Geometry check sheet. Reference: the model listing, model coordinates, mm. A direction names the side the tool comes from. Give positions to 0.01 mm unless a question says otherwise; leave off trailing zeros. Order: outer loops, then holes, each group sorted by start corner. A loop starts at its lowest first (then second) coordinate and runs counter-clockwise, first axis right, second up.
```python
from build123d import *

# Parameters (mm, degrees)
F2_T     = -1
F3_R     = 9.75
F4_DEPTH = 1


with BuildPart() as f1:
    # F0 (on Front) → F1 (revolve)
    with BuildSketch(Plane.XZ):
        Polygon((0, 12), (0, 0), (25, 0), (25, 8), (12.5, 12), align=None)
    revolve(axis=Axis((0, 0, 39.176005), (0, 0, 1)))

    # F2
    f2_openings = [f1.faces().sort_by_distance(p)[0] for p in [
        (0, 0, 0),
    ]]
    offset(amount=F2_T, openings=f2_openings)

    # F3 (on face) → F4 (cut, through all)
    with BuildSketch(Plane.XY.offset(12)):
        Circle(F3_R)
    extrude(amount=-F4_DEPTH, mode=Mode.SUBTRACT)


solid = f1.part
```
Q1. Release check for a two-part mould opening along Y. For faces 1 (the face through (-3.8, -9.2, 12)), 2 (the face through (6, -11.5, 10.8)), 3 (the face through (-10.4, -8, 11.8)) record: pulls with the +Y half, pulls with the -Y half, needs draft (parallel to the pull), parting line crosses it, or undercut.
Q2. Access from +Z, -Z, +X, -X, +Y, -Y to the whole of each face (thin tool, end or side, straight path). Record for faces 4 (the face through (1, 10, 11)), 5 (the face through (9.4, 22.3, 0)).
Q3. Thickness scan on L1, parallel to Y at x = -0.5, z = 1.75 (3 decimals); L2, parallel to Z at x = -11.5, y = 1; L3, parallel to X at y = -14, z = 6. Record the ranges inside material, lowest first.
Q4. Cross-section at C-C, the plane z = 4. Record the boundary of the cut face in (x, y), and give its area (3 significant figures).
Q5. Gauge pin test, flat ends, axial feed: P1, Ø6, axis at x = 3.5, y = -11.5, coming from the -Z side; P2, Ø3, axis at y = 5.5, z = 3, coming from the +X side; P3, Ø5, axis at x = -12.5, y = 13.5, coming from the +Z side; P4, Ø17.5, axis at x = 0, y = 0, coming from the -Z side. Record the tip position at first contact, or that the pin passes through.
Q6. Cross-section at A-A, the plane x = 0. Record the boundary of the cut face in (y, z), and give its area (3 significant figures).
Answers follow:
1. face 1: needs draft
1. face 2: undercut
1. face 3: parting line crosses it
2. face 4: -Z
2. face 5: -Z, +X, -X, +Y, -Y
3. L1: y = -24.995 to -23.995, 23.995 to 24.995
3. L2: z = 11 to 12
3. L3: x = -20.71 to -19.49, 19.49 to 20.71
4. outline: circle Ø50 at (0, 0); hole circle Ø48 at (0, 0)
4. area: 154 mm2
5. P1: stops at z = 10.14
5. P2: stops at x = 24.68
5. P3: stops at z = 10.91
5. P4: passes through
6. outline: (-25, 0) - (-24, 0) - (-24, 7.27) - (-12.34, 11) - (-9.75, 11) - (-9.75, 12) - (-12.5, 12) - (-25, 8) - close; (9.75, 11) - (12.34, 11) - (24, 7.27) - (24, 0) - (25, 0) - (25, 8) - (12.5, 12) - (9.75, 12) - close
6. area: 46.0 mm2
